Can you work these out from the model? Positions are in its coordinate system, mm. A direction names the side the tool comes from. Round coordinates to 2 decimals unless told otherwise and drop trailing zeros. Loops run counter-clockwise (first coordinate to the right, second up) from the corner with the lowest first, then second, coordinate; pieces in that order, holes last. Notation, with made-up numbers: (32.5, -36.75) -> (39.5, -36.75) arc R28 cw to (39.5, -0.75) -> close; hole circle Ø4 at (22, -31). An arc over 180 degrees is marked (long way). Use a Markdown table: item, result.
from build123d import *

# Parameters (mm, degrees)
SKETCH1_W            = 206
SKETCH1_H            = 115
BOSS_EXTRUDE1_DEPTH  = 6.88
SKETCH2_W            = 158
SKETCH2_H            = 95
CUT_EXTRUDE1_DEPTH   = 119.163380114
FILLET1_R            = 10
SKETCH3_W            = 3.55
SKETCH3_H            = 42
CUT_EXTRUDE2_DEPTH   = 119.163380114
SKETCH4_W            = 7.62
SKETCH4_H            = 5
CUT_EXTRUDE3_DEPTH   = 119.163380114
FILLET4_R            = 0.5
SKETCH5_W            = 15
SKETCH5_H            = 6.5
BOSS_EXTRUDE2_DEPTH  = 6.88
FILLET3_R            = 2
FILLET4_OF_MIRROR1_R = 0.5
FILLET3_OF_MIRROR1_R = 2
CUT_EXTRUDE4_START   = -6.88
CUT_EXTRUDE4_DEPTH   = 6.88
SKETCH7_R            = 2.125
SKETCH7_R_2          = 1.524
CUT_EXTRUDE5_DEPTH   = 122.459188207
MIRROR2_START        = -6.88
MIRROR2_OUTLINE_R    = 2.125
MIRROR2_OUTLINE_R_2  = 1.524
MIRROR2_DEPTH        = 6.88
MIRROR2_2_DEPTH      = 6.88
FILLET2_R            = 15


# Read off the part's stored shape, not the designer's step: Cut-Extrude4, Mirror2
with BuildPart() as part:
    # Sketch1 → Boss-Extrude1 (new body)
    with BuildSketch(Plane.XY):
        Rectangle(SKETCH1_W, SKETCH1_H)
    extrude(amount=-BOSS_EXTRUDE1_DEPTH)

    # Sketch2 → Cut-Extrude1 (cut, through all)
    with BuildSketch(Plane.XY):
        Rectangle(SKETCH2_W, SKETCH2_H)
    extrude(amount=-CUT_EXTRUDE1_DEPTH, mode=Mode.SUBTRACT)

    # Fillet1
    fillet1_edges = [part.edges().sort_by_distance(p)[0] for p in [
        (-79, -47.5, -3.44),
        (-79, 47.5, -3.44),
        (79, 47.5, -3.44),
        (79, -47.5, -3.44),
    ]]
    fillet(fillet1_edges, radius=FILLET1_R)

    # Sketch3 → Cut-Extrude2 (cut, through all)
    with BuildSketch(Plane.XY):
        with Locations((-90, 57.5)):
            Rectangle(SKETCH3_W, SKETCH3_H)
    cut_extrude2 = extrude(amount=-CUT_EXTRUDE2_DEPTH, mode=Mode.SUBTRACT)

    # Sketch4 → Cut-Extrude3 (cut, through all)
    with BuildSketch(Plane.XY):
        with Locations((-90, 44)):
            Rectangle(SKETCH4_W, SKETCH4_H)
    cut_extrude3 = extrude(amount=-CUT_EXTRUDE3_DEPTH, mode=Mode.SUBTRACT)

    # Fillet4
    fillet4_edges = [part.edges().sort_by_distance(p)[0] for p in [
        (-88.225, 36.5, -3.44),
        (-91.775, 36.5, -3.44),
        (-86.19, 41.5, -3.44),
        (-93.81, 46.5, -3.44),
        (-86.19, 46.5, -3.44),
        (-93.81, 41.5, -3.44),
    ]]
    fillet(fillet4_edges, radius=FILLET4_R)

    # Sketch5 → Boss-Extrude2 (add)
    with BuildSketch(Plane.XY):
        with Locations((-57.5, 60.75)):
            Rectangle(SKETCH5_W, SKETCH5_H)
    boss_extrude2 = extrude(amount=-BOSS_EXTRUDE2_DEPTH)

    # Fillet3
    fillet3_edges = [part.edges().sort_by_distance(p)[0] for p in [
        (-50, 64, -3.44),
        (-65, 64, -3.44),
    ]]
    fillet(fillet3_edges, radius=FILLET3_R)

    # Mirror1: Cut-Extrude2, Cut-Extrude3, Boss-Extrude2 across plane
    add(cut_extrude2.mirror(Plane.ZX), mode=Mode.SUBTRACT)
    add(cut_extrude3.mirror(Plane.ZX), mode=Mode.SUBTRACT)
    add(boss_extrude2.mirror(Plane.ZX))

    # Fillet4 of Mirror1
    fillet4_of_mirror1_edges = [part.edges().sort_by_distance(p)[0] for p in [
        (-88.225, -36.5, -3.44),
        (-91.775, -36.5, -3.44),
        (-86.19, -41.5, -3.44),
        (-93.81, -46.5, -3.44),
        (-86.19, -46.5, -3.44),
        (-93.81, -41.5, -3.44),
    ]]
    fillet(fillet4_of_mirror1_edges, radius=FILLET4_OF_MIRROR1_R)

    # Fillet3 of Mirror1
    fillet3_of_mirror1_edges = [part.edges().sort_by_distance(p)[0] for p in [
        (-50, -64, -3.44),
        (-65, -64, -3.44),
    ]]
    fillet(fillet3_of_mirror1_edges, radius=FILLET3_OF_MIRROR1_R)

    # Cut-Extrude4 outline → Cut-Extrude4 (cut)
    with BuildSketch(Plane.XY.offset(CUT_EXTRUDE4_START)):
        with BuildLine():
            Line((-78.396926208, 40.920201433), (-86, 20.030927871))
            Line((-86, 20.030927871), (-86, -20.030927871))
            Line((-86, -20.030927871), (-78.396926208, -40.920201433))
            ThreePointArc((-78.396926208, -40.920201433), (-78.84807753, -39.236481777), (-79, -37.5))
            Line((-79, -37.5), (-79, 37.5))
            ThreePointArc((-79, 37.5), (-78.84807753, 39.236481777), (-78.396926208, 40.920201433))
        make_face()
    extrude(amount=CUT_EXTRUDE4_DEPTH, mode=Mode.SUBTRACT)

    # Sketch7 → Cut-Extrude5 (cut, through all)
    with BuildSketch(Plane.XY):
        with Locations((-92, 25)):
            Circle(SKETCH7_R)
        with Locations((-92, -25)):
            Circle(SKETCH7_R)
        with Locations((-96, 0)):
            Circle(SKETCH7_R_2)
    extrude(amount=-CUT_EXTRUDE5_DEPTH, mode=Mode.SUBTRACT)

    # Mirror2 outline → Mirror2 (cut)
    with BuildSketch(Plane.XY.offset(MIRROR2_START)):
        with BuildLine():
            Line((88.225, 57.5), (88.225, 46.5))
            Line((88.225, 46.5), (86.69, 46.5))
            ThreePointArc((86.69, 46.5), (86.336446609, 46.353553391), (86.19, 46))
            Line((86.19, 46), (86.19, 42))
            ThreePointArc((86.19, 42), (86.336446609, 41.646446609), (86.69, 41.5))
            Line((86.69, 41.5), (88.225, 41.5))
            Line((88.225, 41.5), (88.225, 37))
            ThreePointArc((88.225, 37), (88.371446609, 36.646446609), (88.725, 36.5))
            Line((88.725, 36.5), (91.275, 36.5))
            ThreePointArc((91.275, 36.5), (91.628553391, 36.646446609), (91.775, 37))
            Line((91.775, 37), (91.775, 41.5))
            Line((91.775, 41.5), (93.31, 41.5))
            ThreePointArc((93.31, 41.5), (93.663553391, 41.646446609), (93.81, 42))
            Line((93.81, 42), (93.81, 46))
            ThreePointArc((93.81, 46), (93.663553391, 46.353553391), (93.31, 46.5))
            Line((93.31, 46.5), (91.775, 46.5))
            Line((91.775, 46.5), (91.775, 57.5))
            Line((91.775, 57.5), (88.225, 57.5))
        make_face()
        with BuildLine():
            ThreePointArc((88.725, -36.5), (88.371446609, -36.646446609), (88.225, -37))
            Line((88.225, -37), (88.225, -41.5))
            Line((88.225, -41.5), (86.69, -41.5))
            ThreePointArc((86.69, -41.5), (86.336446609, -41.646446609), (86.19, -42))
            Line((86.19, -42), (86.19, -46))
            ThreePointArc((86.19, -46), (86.336446609, -46.353553391), (86.69, -46.5))
            Line((86.69, -46.5), (88.225, -46.5))
            Line((88.225, -46.5), (88.225, -57.5))
            Line((88.225, -57.5), (91.775, -57.5))
            Line((91.775, -57.5), (91.775, -46.5))
            Line((91.775, -46.5), (93.31, -46.5))
            ThreePointArc((93.31, -46.5), (93.663553391, -46.353553391), (93.81, -46))
            Line((93.81, -46), (93.81, -42))
            ThreePointArc((93.81, -42), (93.663553391, -41.646446609), (93.31, -41.5))
            Line((93.31, -41.5), (91.775, -41.5))
            Line((91.775, -41.5), (91.775, -37))
            ThreePointArc((91.775, -37), (91.628553391, -36.646446609), (91.275, -36.5))
            Line((91.275, -36.5), (88.725, -36.5))
        make_face()
        with BuildLine():
            Line((86, -20.030927871), (86, 20.030927871))
            Line((86, 20.030927871), (78.396926208, 40.920201433))
            ThreePointArc((78.396926208, 40.920201433), (78.84807753, 39.236481777), (79, 37.5))
            Line((79, 37.5), (79, -37.5))
            ThreePointArc((79, -37.5), (78.84807753, -39.236481777), (78.396926208, -40.920201433))
            Line((78.396926208, -40.920201433), (86, -20.030927871))
        make_face()
        with Locations((92, 25)):
            Circle(MIRROR2_OUTLINE_R)
        with Locations((92, -25)):
            Circle(MIRROR2_OUTLINE_R)
        with Locations((96, 0)):
            Circle(MIRROR2_OUTLINE_R_2)
    extrude(amount=MIRROR2_DEPTH, mode=Mode.SUBTRACT)

    # Mirror2 2 outline → Mirror2 2 (add)
    with BuildSketch(Plane.XY.offset(MIRROR2_START)):
        with BuildLine():
            Line((50, 57.5), (65, 57.5))
            Line((65, 57.5), (65, 62))
            ThreePointArc((65, 62), (64.414213562, 63.414213562), (63, 64))
            Line((63, 64), (52, 64))
            ThreePointArc((52, 64), (50.585786438, 63.414213562), (50, 62))
            Line((50, 62), (50, 57.5))
        make_face()
        with BuildLine():
            Line((65, -62), (65, -57.5))
            Line((65, -57.5), (50, -57.5))
            Line((50, -57.5), (50, -62))
            ThreePointArc((50, -62), (50.585786438, -63.414213562), (52, -64))
            Line((52, -64), (63, -64))
            ThreePointArc((63, -64), (64.414213562, -63.414213562), (65, -62))
        make_face()
    extrude(amount=MIRROR2_2_DEPTH)

    # Fillet2
    fillet2_edges = [part.edges().sort_by_distance(p)[0] for p in [
        (-86, -20.030927871, -3.44),
        (-86, 20.030927871, -3.44),
        (86, 20.030927871, -3.44),
        (86, -20.030927871, -3.44),
    ]]
    fillet(fillet2_edges, radius=FILLET2_R)


solid = part.part
1. Which directions (+Z, -Z, +X, -X, +Y, -Y) give clear straight access to the entire face, cutting with the end or side of a thin tool? Please do faces 1 (the flat face through (-77, 57.5, -3)), 2 (the flat face through (-81.793, -31.589, -3.488)), 3 (the flat face through (-50, -60, -3)), 4 (the flat face through (-91.775, 52, -3)), 5 (the flat face through (-65, -60, -3)).
Answer sheet:
| item | result |
|---|---|
| face 1 | +Z, -Z, -X, +Y |
| face 2 | +Z, -Z |
| face 3 | +Z, -Z, -Y |
| face 4 | +Z, -Z, +Y |
| face 5 | +Z, -Z, -X, -Y |
2. I need wall thicknesses on line 1 (Y direction, x = 87.5, z = -3); line 2 (Y direction, x = 92, z = -4) (3 decimals); line 3 (X direction, y = -54, z = -2.5) (3 decimals). Which ranges of each line are inside material? Lowest first, please.
Answer sheet:
| item | result |
|---|---|
| line 1 | y = -57.5 to -46.5, -41.5 to 41.5, 46.5 to 57.5 |
| line 2 | y = -57.5 to -46.5, -41.5 to -27.125, -22.875 to 22.875, 27.125 to 41.5, 46.5 to 57.5 |
| line 3 | x = -103 to -91.775, -88.225 to 88.225, 91.775 to 103 |
3. I want a section at B-B (x = 27.5). Please give me the cut outline in (y, z), plus the area to 3 significant figures.
Answer sheet:
| item | result |
|---|---|
| outline | (-57.5, -6.88) -> (-47.5, -6.88) -> (-47.5, 0) -> (-57.5, 0) -> close; (47.5, -6.88) -> (57.5, -6.88) -> (57.5, 0) -> (47.5, 0) -> close |
| area | 138 mm² |
4. I want a section at C-C (y = -25). Please give me the cut outline in (x, z) (3 decimals).
Answer sheet:
| item | result |
|---|---|
| outline | (-103, -6.88) -> (-94.125, -6.88) -> (-94.125, 0) -> (-103, 0) -> close; (-89.875, -6.88) -> (-84.191, -6.88) -> (-84.191, 0) -> (-89.875, 0) -> close; (84.191, -6.88) -> (89.875, -6.88) -> (89.875, 0) -> (84.191, 0) -> close; (94.125, -6.88) -> (103, -6.88) -> (103, 0) -> (94.125, 0) -> close |
5. I want a section at A-A (y = 15). Please give me the cut outline in (x, z).
Answer sheet:
| item | result |
|---|---|
| outline | (-103, -6.88) -> (-86, -6.88) -> (-86, 0) -> (-103, 0) -> close; (86, -6.88) -> (103, -6.88) -> (103, 0) -> (86, 0) -> close |
6. If we mould it in two halves opening along X, with no side actions, what happens to faces 6 (the flat face through (-93.81, 44, -3)), 7 (the flat face through (-65, 60, -3)), 8 (the flat face through (-77, -57.5, -3))? For each: +X half, -X half, draft (parallel to the pull), parting line (faces both ways), or undercut.
Answer sheet:
| item | result |
|---|---|
| face 6 | undercut |
| face 7 | -X half |
| face 8 | draft |
7. Will these pins go through, and if not, where does the flat tip stop? pin 1 Ø0.8 at (x, z) = (87, -3.5) entering from -Y; pin 2 Ø3.5 at (x, y) = (92, -25) entering from -Z; pin 3 Ø1 at (x, z) = (-5, -2) entering from +Y; pin 4 Ø3.5 at (y, z) = (-60.5, -2.5) entering from +X.
Answer sheet:
| item | result |
|---|---|
| pin 1 | stops at y = -57.5 |
| pin 2 | passes through |
| pin 3 | stops at y = 57.5 |
| pin 4 | stops at x = 65 |
8. I want a section at D-D (z = -3.5). State how many separate pieces and enclosed holes the cut face has, plus the area to 3 significant figures.
Answer sheet:
| item | result |
|---|---|
| separate pieces | 1 |
| enclosed holes | 7 |
| area | 7,870 mm² |
